The listing builds one solid part. Answer for the finished solid, in the listing's coordinates (mm). A direction names the side the tool comes from. Give positions to 0.01 mm unless a question says otherwise; leave off trailing zeros. Loops run counter-clockwise (first coordinate to the right, second up) from the corner with the lowest first, then second, coordinate; pieces in that order, holes last. Notation, with made-up numbers: M -19,56 L -8,56 A20 cw -8,68 Z; hole C -20,-22.75 d10. An arc over 180 degrees is marked long. Use one line per item in the form item = value. Start each with the question number.
1. The mould has two halves that part along Z. Classify faces 4 (the face through (57, 8, 12)), 5 (the face through (57, 8, 2)), 6 (the face through (104, 6, 65)), 7 (the face through (58, 8, 0)): released by +Z, released by -Z, zero draft, split by the parting line, or undercut.
2. The part is cut by section B-B (z = 60). Write down the section's boundary in (x, y), and give its area (3 significant figures).
3. The part is cut by section C-C (y = 6.5). Write down the section's boundary in (x, z).
4. Each of these flat-tipped pins is pushed along its axis until it touches: pin 1 Ø3 at (y, z) = (3.5, 75) entering from -X; pin 2 Ø7 at (y, z) = (6.5, 49.5) entering from +X; pin 3 Ø6.5 at (x, z) = (52, 6) entering from -Y. Where does it stop, or does it pass through?
5. For faces 1 (the face through (109, 2, 65)), 2 (the face through (2, 7, 6)), 3 (the face through (102, 1, 6)), determine the directions among +Z, -Z, +X, -X, +Y, -Y from which every point of the face is accessible in a straight line to the end or side of a thin tool.
6. Straight lines are drawn through the part: line 1 (Z direction, x = 61.5, y = 7.75); line 2 (Z direction, x = 103, y = 7.5); line 3 (Y direction, x = 108, z = 63). For each, find the intervals that lie inside material, in ascending order. Write a range as from..to.
7. The part is cut by section A-A (x = 87.5). Write down the section's boundary in (y, z), and give its area (3 significant figures).
from build123d import *

# Parameters (mm, degrees)
BOSS_EXTRUDE1_DEPTH = 2
BOSS_EXTRUDE2_DEPTH = 11
SKETCH3_W           = 9
SKETCH3_H           = 9
CUT_EXTRUDE1_DEPTH  = 2
BOSS_EXTRUDE3_DEPTH = 109
BOSS_EXTRUDE4_DEPTH = 1
FILLET1_R           = 2


with BuildPart() as part:
    # Sketch1 → Boss-Extrude1 (new body)
    with BuildSketch(Plane(origin=(0, 0, 0), x_dir=(1, 0, 0), z_dir=(0, 1, 0))):
        Polygon((0, 0), (0, -12), (113, -12), (113, -10), (102, -10), (102, -2), (113, -2), (113, 0), align=None)
    extrude(amount=BOSS_EXTRUDE1_DEPTH)

    # Sketch2 → Boss-Extrude2 (add)
    with BuildSketch(Plane(origin=(0, 2, 0), x_dir=(1, 0, 0), z_dir=(0, 1, 0))):
        Polygon((2, -10), (2, -2), (102, -2), (113, -2), (113, 0), (0, 0), (0, -12), (113, -12), (113, -10), (102, -10), align=None)
    extrude(amount=BOSS_EXTRUDE2_DEPTH)

    # Sketch3 → Cut-Extrude1 (cut)
    with BuildSketch(Plane.XY.offset(12)):
        with Locations((108.5, 6.5)):
            Rectangle(SKETCH3_W, SKETCH3_H)
    extrude(amount=-CUT_EXTRUDE1_DEPTH, mode=Mode.SUBTRACT)

    # Sketch3<3> → Boss-Extrude3 (add)
    with BuildSketch(Plane.XY.offset(12)):
        Polygon((113, 0), (113, 2), (104, 2), (104, 11), (113, 11), (113, 13), (102, 13), (102, 0), align=None)
    extrude(amount=BOSS_EXTRUDE3_DEPTH)

    # Sketch1<3> → Boss-Extrude4 (add)
    with BuildSketch(Plane(origin=(0, 0, 0), x_dir=(1, 0, 0), z_dir=(0, 1, 0))):
        Polygon((113, 0), (100, 0), (100, -12), (113, -12), (113, -10), (102, -10), (102, -2), (113, -2), align=None)
    extrude(amount=-BOSS_EXTRUDE4_DEPTH)

    # Fillet1
    fillet1_edges = [part.edges().sort_by_distance(p)[0] for p in [
        (100, -0.5, 0),
        (50, 0, 12),
        (0, 0, 6),
        (50, 0, 0),
        (0, 6.5, 12),
        (0, 6.5, 0),
        (102, 0, 66.5),
        (100, -0.5, 12),
    ]]
    fillet(fillet1_edges, radius=FILLET1_R - 0.0001)  # a hair under: the kernel refuses the full size


solid = part.part
Derived:
q1.face_4 = released by +Z
q1.face_5 = undercut
q1.face_6 = zero draft
q1.face_7 = released by -Z
q2.outline = M 102,2 A2 ccw 104,0 L 113,0 L 113,2 L 104,2 L 104,11 L 113,11 L 113,13 L 102,13 Z
q2.area = 61.1 mm2
q3.outline = M 0,2 A2 ccw 2,0 L 113,0 L 113,2 L 2,2 L 2,10 L 104,10 L 104,121 L 102,121 L 102,12 L 2,12 A2 ccw 0,10 Z
q4.pin_1 = 102
q4.pin_2 = 104
q4.pin_3 = 0
q5.face_1 = +Z, +X
q5.face_2 = +X, +Y
q5.face_3 = +X, +Y, -Y
q6.line_1 = 0..2, 10..12
q6.line_2 = 0..2, 10..121
q6.line_3 = 0..2, 11..13
q7.outline = M 0,2 A2 ccw 2,0 L 13,0 L 13,2 L 2,2 L 2,10 L 13,10 L 13,12 L 2,12 A2 ccw 0,10 Z
q7.area = 66.3 mm2
